Geometry: final body of the model. Coordinates: model frame, mm. Face numbers are marked on the shaded views. A direction names the side the tool comes from. Give positions to 0.01 mm unless a question says otherwise; leave off trailing zeros. Order: outer loops, then holes, each group sorted by start corner. A loop starts at its lowest first (then second) coordinate and runs counter-clockwise, first axis right, second up. Notation, with made-up numbers: M -11.5,-18.75 L 36.5,-18.75 A17 ccw 36.5,-10.75 Z; hole C 27,15 d11. An arc over 180 degrees is marked long. Write item = value, one per line. Start each with the question number.
from build123d import *

# Parameters (mm, degrees)
F1_DEPTH     = 25
F2_R         = 2.5
F3_DEPTH     = 46.9
F4_T1_DEPTH  = 150
F4_T3_DEPTH  = 182.2274848408
F4_T5_DEPTH  = 100.3173754326
F4_T10_DEPTH = 75.5924176596
F4_T15_DEPTH = 87.245278787
F4_T20_DEPTH = 99.0010747165
F4_T25_DEPTH = 85.6788355908
F4_T30_DEPTH = 82.646426835
F4_T35_DEPTH = 119.0871070802
F4_T41_DEPTH = 75.5924176596
F4_T45_DEPTH = 87.245278787
F4_T52_DEPTH = 85.6788355908
F4_T56_DEPTH = 99.0010747165
F4_T63_DEPTH = 119.0871070802
F4_T67_DEPTH = 82.646426835


# Not quite as in the source:
# - a fillet or chamfer that OpenCascade refuses, or shapes differently, is made with other operations: its cross-section is extruded or revolved along the edge and cut away or added


with BuildPart() as f1:
    # F0 (on Front) → F1 (new body)
    with BuildSketch(Plane.XZ):
        Polygon((49.0980417262, 68.0754659733), (-83.1294431146, 68.0754659733), (-83.1294431146, -31.9245340267), (-32.8924826343, -34.7681359889), (-32.8924826343, -9.1757183293), (3.1264783981, -18.6543911301), (-25.4433550304, 21.1560339021), (10.2354805604, 21.1560339021), (-14.8830008989, 42.00911699), align=None)
    extrude(amount=F1_DEPTH)

    # F2 (on Front) → F3 (cut)
    with BuildSketch(Plane.XZ):
        with Locations((-80.3935006261, 58.4694631398)):
            Circle(F2_R)
    extrude(amount=F3_DEPTH, mode=Mode.SUBTRACT)

    # F4: fillet of radius 10 on 9 edges, made by hand

    # F4_s2 → F4_t1 (cut)
    with BuildSketch(Plane.XY.offset(-56.9245340267)):
        with BuildLine():
            ThreePointArc((-83.1294431146, -10), (-80.2005109264, -2.9289321881), (-73.1294431146, 0))
            Line((-73.1294431146, 0), (-83.1294431146, 0))
            Line((-83.1294431146, 0), (-83.1294431146, -10))
        make_face()
    extrude(amount=F4_T1_DEPTH, mode=Mode.SUBTRACT)

    # F4_s4 → F4_t3 (cut)
    with BuildSketch(Plane.YZ.offset(-108.1294431146)):
        with BuildLine():
            ThreePointArc((-10, 68.0754659733), (-2.9289321881, 65.1465337851), (0, 58.0754659733))
            Line((0, 58.0754659733), (0, 68.0754659733))
            Line((0, 68.0754659733), (-10, 68.0754659733))
        make_face()
    extrude(amount=F4_T3_DEPTH, mode=Mode.SUBTRACT)

    # F4_s6 → F4_t5 (cut)
    with BuildSketch(Plane(origin=(-106.0227160465, 0, 6.0012867121), x_dir=(0, 1, 0), z_dir=(0.9984018453, 0, -0.0565133205))):
        with BuildLine():
            ThreePointArc((0, -26.5714345391), (-2.9289321881, -33.6425023509), (-10, -36.5714345391))
            Line((-10, -36.5714345391), (0, -36.5714345391))
            Line((0, -36.5714345391), (0, -26.5714345391))
        make_face()
    extrude(amount=F4_T5_DEPTH, mode=Mode.SUBTRACT)


with BuildPart() as f4_tool8:
    # F4_s9 → F4_t10 (new body)
    with BuildSketch(Plane.XY.offset(-59.7681359889)):
        with BuildLine():
            ThreePointArc((-42.8924826343, 0), (-35.8214148224, -2.9289321881), (-32.8924826343, -10))
            Line((-32.8924826343, -10), (-32.8924826343, 0))
            Line((-32.8924826343, 0), (-42.8924826343, 0))
        make_face()
    extrude(amount=F4_T10_DEPTH)

    split(bisect_by=Plane(origin=(-4.3886140602, 0, -16.676735461), x_dir=(0, 1, 0), z_dir=(-0.2544932703, 0, -0.9670745449)), keep=Keep.TOP)


with BuildPart() as f1_1:
    add(f1.part)

    # F4_t7: cut F4_tool8
    add(f4_tool8.part, mode=Mode.SUBTRACT)


with BuildPart() as f4_tool13:
    # F4_s14 → F4_t15 (new body)
    with BuildSketch(Plane(origin=(-52.6807321964, 0, 13.8633488887), x_dir=(0, 1, 0), z_dir=(0.9670745449, 0, -0.2544932703))):
        with BuildLine():
            ThreePointArc((0, -7.2445191005), (-2.9289321881, -14.3155869123), (-10, -17.2445191005))
            Line((-10, -17.2445191005), (0, -17.2445191005))
            Line((0, -17.2445191005), (0, -7.2445191005))
        make_face()
    extrude(amount=F4_T15_DEPTH)

    split(bisect_by=Plane.YZ.offset(-32.8924826343), keep=Keep.TOP)


with BuildPart() as f1_2:
    add(f1_1.part)

    # F4_t12: cut F4_tool13
    add(f4_tool13.part, mode=Mode.SUBTRACT)


with BuildPart() as f4_tool18:
    # F4_s19 → F4_t20 (new body)
    with BuildSketch(Plane(origin=(24.4753258646, 0, -34.1049634717), x_dir=(0, 1, 0), z_dir=(-0.5830450371, 0, 0.8124398345))):
        with BuildLine():
            ThreePointArc((0, 18.3362745772), (-2.9289321881, 11.2652067653), (-10, 8.3362745772))
            Line((-10, 8.3362745772), (0, 8.3362745772))
            Line((0, 8.3362745772), (0, 18.3362745772))
        make_face()
    extrude(amount=F4_T20_DEPTH)

    split(bisect_by=Plane.XY.offset(21.1560339021), keep=Keep.BOTTOM)


with BuildPart() as f1_3:
    add(f1_2.part)

    # F4_t17: cut F4_tool18
    add(f4_tool18.part, mode=Mode.SUBTRACT)


with BuildPart() as f4_tool23:
    # F4_s24 → F4_t25 (new body)
    with BuildSketch(Plane.YZ.offset(-50.4433550304)):
        with BuildLine():
            ThreePointArc((0, 31.1560339021), (-2.9289321881, 24.0849660902), (-10, 21.1560339021))
            Line((-10, 21.1560339021), (0, 21.1560339021))
            Line((0, 21.1560339021), (0, 31.1560339021))
        make_face()
    extrude(amount=F4_T25_DEPTH)

    split(bisect_by=Plane(origin=(-6.7727215377, 0, -4.8604235206), x_dir=(0, 1, 0), z_dir=(0.8124398345, 0, 0.5830450371)), keep=Keep.TOP)


with BuildPart() as f1_4:
    add(f1_3.part)

    # F4_t22: cut F4_tool23
    add(f4_tool23.part, mode=Mode.SUBTRACT)


with BuildPart() as f4_tool28:
    # F4_s29 → F4_t30 (new body)
    with BuildSketch(Plane(origin=(14.897118547, 0, -12.3674216268), x_dir=(0, 1, 0), z_dir=(-0.769409822, 0, 0.6387554507))):
        with BuildLine():
            ThreePointArc((0, -12.8156292772), (-2.9289321881, -19.8866970891), (-10, -22.8156292772))
            Line((-10, -22.8156292772), (0, -22.8156292772))
            Line((0, -22.8156292772), (0, -12.8156292772))
        make_face()
    extrude(amount=F4_T30_DEPTH)

    split(bisect_by=Plane(origin=(-16.7971177223, 0, 41.2292916688), x_dir=(0, 1, 0), z_dir=(0.377296866, 0, -0.9260923684)), keep=Keep.TOP)


with BuildPart() as f1_5:
    add(f1_4.part)

    # F4_t27: cut F4_tool28
    add(f4_tool28.part, mode=Mode.SUBTRACT)


with BuildPart() as f4_tool33:
    # F4_s34 → F4_t35 (new body)
    with BuildSketch(Plane(origin=(-21.2381923878, 0, -8.6525963291), x_dir=(0, 1, 0), z_dir=(0.9260923684, 0, 0.377296866))):
        with BuildLine():
            ThreePointArc((-10, 44.5196322457), (-2.9289321881, 47.4485644338), (0, 54.5196322457))
            Line((0, 54.5196322457), (0, 44.5196322457))
            Line((0, 44.5196322457), (-10, 44.5196322457))
        make_face()
    extrude(amount=F4_T35_DEPTH)

    split(bisect_by=Plane(origin=(14.5736075628, 0, 17.5545692605), x_dir=(0, 1, 0), z_dir=(0.6387554507, 0, 0.769409822)), keep=Keep.TOP)


with BuildPart() as f1_6:
    add(f1_5.part)

    # F4_t32: cut F4_tool33
    add(f4_tool33.part, mode=Mode.SUBTRACT)


with BuildPart() as f4_tool39:
    # F4_s40 → F4_t41 (new body)
    with BuildSketch(Plane.XY.offset(-59.7681359889)):
        with BuildLine():
            ThreePointArc((-42.8924826343, 0), (-35.8214148224, -2.9289321881), (-32.8924826343, -10))
            Line((-32.8924826343, -10), (-32.8924826343, 0))
            Line((-32.8924826343, 0), (-42.8924826343, 0))
        make_face()
    extrude(amount=F4_T41_DEPTH)

    split(bisect_by=Plane(origin=(-4.3886140602, 0, -16.676735461), x_dir=(0, 1, 0), z_dir=(0.2544932703, 0, 0.9670745449)), keep=Keep.TOP)


with BuildPart() as f4_tool43:
    # F4_s44 → F4_t45 (new body)
    with BuildSketch(Plane(origin=(-52.6807321964, 0, 13.8633488887), x_dir=(0, 1, 0), z_dir=(0.9670745449, 0, -0.2544932703))):
        with BuildLine():
            ThreePointArc((0, -7.2445191005), (-2.9289321881, -14.3155869123), (-10, -17.2445191005))
            Line((-10, -17.2445191005), (0, -17.2445191005))
            Line((0, -17.2445191005), (0, -7.2445191005))
        make_face()
    extrude(amount=F4_T45_DEPTH)

    split(bisect_by=Plane.YZ.offset(-32.8924826343), keep=Keep.BOTTOM)


with BuildPart() as f4_tool39_1:
    add(f4_tool39.part)

    # F4_t47: intersect F4_tool43
    add(f4_tool43.part, mode=Mode.INTERSECT)


with BuildPart() as f1_7:
    add(f1_6.part)

    # F4_t37: cut F4_tool39
    add(f4_tool39_1.part, mode=Mode.SUBTRACT)


with BuildPart() as f4_tool50:
    # F4_s51 → F4_t52 (new body)
    with BuildSketch(Plane.YZ.offset(-50.4433550304)):
        with BuildLine():
            ThreePointArc((0, 31.1560339021), (-2.9289321881, 24.0849660902), (-10, 21.1560339021))
            Line((-10, 21.1560339021), (0, 21.1560339021))
            Line((0, 21.1560339021), (0, 31.1560339021))
        make_face()
    extrude(amount=F4_T52_DEPTH)

    split(bisect_by=Plane(origin=(-6.7727215377, 0, -4.8604235206), x_dir=(0, 1, 0), z_dir=(-0.8124398345, 0, -0.5830450371)), keep=Keep.TOP)


with BuildPart() as f4_tool54:
    # F4_s55 → F4_t56 (new body)
    with BuildSketch(Plane(origin=(24.4753258646, 0, -34.1049634717), x_dir=(0, 1, 0), z_dir=(-0.5830450371, 0, 0.8124398345))):
        with BuildLine():
            ThreePointArc((0, 18.3362745772), (-2.9289321881, 11.2652067653), (-10, 8.3362745772))
            Line((-10, 8.3362745772), (0, 8.3362745772))
            Line((0, 8.3362745772), (0, 18.3362745772))
        make_face()
    extrude(amount=F4_T56_DEPTH)

    split(bisect_by=Plane.XY.offset(21.1560339021), keep=Keep.TOP)


with BuildPart() as f4_tool50_1:
    add(f4_tool50.part)

    # F4_t58: intersect F4_tool54
    add(f4_tool54.part, mode=Mode.INTERSECT)


with BuildPart() as f1_8:
    add(f1_7.part)

    # F4_t48: cut F4_tool50
    add(f4_tool50_1.part, mode=Mode.SUBTRACT)


with BuildPart() as f4_tool61:
    # F4_s62 → F4_t63 (new body)
    with BuildSketch(Plane(origin=(-21.2381923878, 0, -8.6525963291), x_dir=(0, 1, 0), z_dir=(0.9260923684, 0, 0.377296866))):
        with BuildLine():
            ThreePointArc((-10, 44.5196322457), (-2.9289321881, 47.4485644338), (0, 54.5196322457))
            Line((0, 54.5196322457), (0, 44.5196322457))
            Line((0, 44.5196322457), (-10, 44.5196322457))
        make_face()
    extrude(amount=F4_T63_DEPTH)

    split(bisect_by=Plane(origin=(14.5736075628, 0, 17.5545692605), x_dir=(0, 1, 0), z_dir=(-0.6387554507, 0, -0.769409822)), keep=Keep.TOP)


with BuildPart() as f4_tool65:
    # F4_s66 → F4_t67 (new body)
    with BuildSketch(Plane(origin=(14.897118547, 0, -12.3674216268), x_dir=(0, 1, 0), z_dir=(-0.769409822, 0, 0.6387554507))):
        with BuildLine():
            ThreePointArc((0, -12.8156292772), (-2.9289321881, -19.8866970891), (-10, -22.8156292772))
            Line((-10, -22.8156292772), (0, -22.8156292772))
            Line((0, -22.8156292772), (0, -12.8156292772))
        make_face()
    extrude(amount=F4_T67_DEPTH)

    split(bisect_by=Plane(origin=(-16.7971177223, 0, 41.2292916688), x_dir=(0, 1, 0), z_dir=(-0.377296866, 0, 0.9260923684)), keep=Keep.TOP)


with BuildPart() as f4_tool61_1:
    add(f4_tool61.part)

    # F4_t69: intersect F4_tool65
    add(f4_tool65.part, mode=Mode.INTERSECT)


with BuildPart() as f1_9:
    add(f1_8.part)

    # F4_t59: cut F4_tool61
    add(f4_tool61_1.part, mode=Mode.SUBTRACT)


solid = f1_9.part
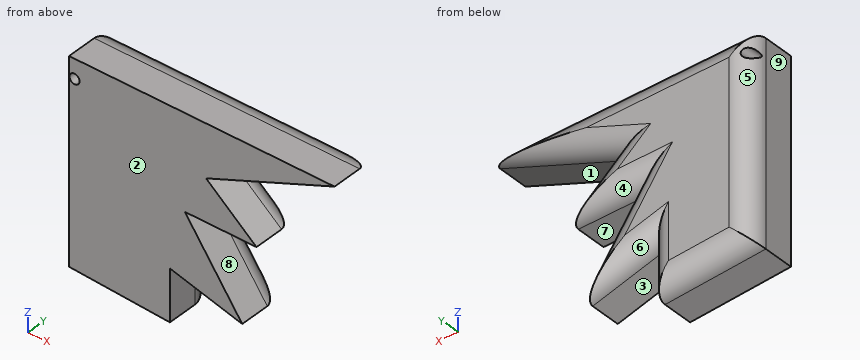
1) Ray query, L1, parallel to Z at x = -4, y = -15.5; L2, parallel to Z at x = 1, y = -21.25; L3, parallel to Z at x = -16, y = -9. Return the intervals inside material, ascending.
2) Access query for the marked faces 1, 2, 3, 4 and 5. Directions: +Z, -Z, +X, -X, +Y, -Y. A direction counts if a zero-diameter tool reaches every point of the face in a straight line with its end or side. Return the directions, or none.
3) Cut plane A-A (y = -20.25). Return loops of the section in (x, z).
4) Pin query (flat end, axial travel): pin 1 Ø6.5 at (x, z) = (-80.39, 58.47) entering from +Y; pin 2 Ø4 at (y, z) = (-12.5, 51.5) entering from +X; pin 3 Ø7.5 at (x, y) = (-6, -15) entering from -Z. Return the tip coordinate at first contact, or that it passes through.
5) Draft query along Z for the marked faces 6, 7, 8 and 9. Return one class per face: pulls with the +Z half, pulls with the -Z half, needs draft (parallel to the pull), parting line crosses it, or undercut.
6) Cut plane B-B (y = -6.25). Return loops of the section in (x, z).
Reply:
q1.L1 = -16.78 to -8.72, 21.16 to 32.97, 46.44 to 68.08
q1.L2 = -18.09 to -15.69, 21.16 to 28.82, 48.48 to 68.08
q1.L3 = -13.57 to 7.91, 21.21 to 68.03
q2.face_1 = +X, +Y, -Y
q2.face_2 = +Z, -Z, +X, -X, -Y
q2.face_3 = -Z, +Y, -Y
q2.face_4 = +X, +Y
q2.face_5 = +Z, -Z, -X, +Y
q3.outline = M -83.13,-31.92 L -32.89,-34.77 L -32.89,-9.18 L 3.13,-18.65 L -25.44,21.16 L 10.24,21.16 L -14.88,42.01 L 49.1,68.08 L -83.13,68.08 Z; hole C -80.39,58.47 d5
q4.pin_1 = -0.84
q4.pin_2 = 13.32
q4.pin_3 = -17.24
q5.face_6 = pulls with the -Z half
q5.face_7 = undercut
q5.face_8 = undercut
q5.face_9 = needs draft
q6.outline = M -82.4,-31.23 L -33.62,-34 L -33.62,-8.23 L 1.35,-17.43 L -26.87,21.89 L 8.21,21.89 L -16.29,42.23 L 45.37,67.35 L -82.4,67.35 L -82.4,59.96 A2.5 cw long -82.4,56.98 Z
